Job drawing, mm, ordinate dimensions from the low corner. One solid piece. A direction names the side the tool comes from. Give positions to 0.01 mm unless a question says otherwise; leave off trailing zeros. Order: outer loops, then holes, each group sorted by start corner. A loop starts at its lowest first (then second) coordinate and runs counter-clockwise, first axis right, second up. Notation, with made-up numbers: (-5, 39) - (-1, 39) arc R18 cw to (-1, 69) - close; hole circle Ø10 at (87, -20). An arc over 180 degrees is marked (long way). Write each question's results on one line, items separated by ' | '. Start each with the question number.
1) Drop a flat-ended pin along its axis: pin 1 Ø2.5 at (x, y) = (4.5, 8.5) entering from +Z. Give the stop position or say it passes through.
2) Cut at D-D on y = 6.25. List the corners of the cut face in (x, z) (1 decimal).
3) Cut at A-A on x = 4.25. List the corners of the cut face in (y, z), plus the area to 3 significant figures.
4) Cut at C-C on z = 3.5. List the corners of the cut face in (x, y), plus the area to 3 significant figures.
5) Two-plate mould, pull along Y, no slides. Class the marked faces 3, 4, 5 and 6: +Y half, -Y half, draft (parallel to the pull), parting line (faces both ways), or undercut.
6) Tool access for the marked faces 1 and 2: list every direction of +Z, -Z, +X, -X, +Y, -Y with a clear straight run to the whole face (end or side of a thin tool).
7) Drill centre lines: line 1 along Z through (x, y) = (1.5, 2.25); line 2 along Y through (x, z) = (5.25, 10.25) (1 decimal); line 3 along X through (y, z) = (8.75, 4) (1 decimal). Where is each one in solid material? Low to high. Write a range as from..to.
8) Cut at B-B on y = 10.5. List the corners of the cut face in (x, z) (1 decimal).
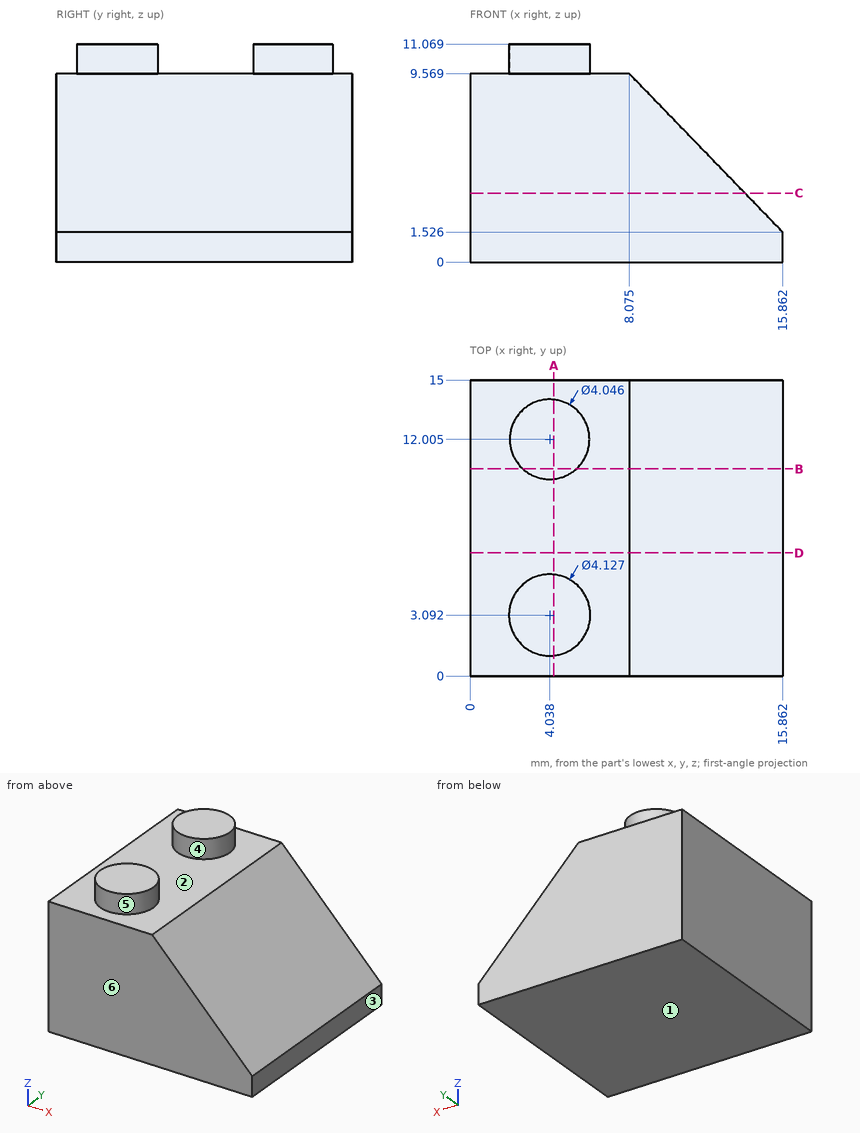
Results:
1) pin 1: z = 9.57
2) outline: (0, 0) - (15.9, 0) - (15.9, 1.5) - (8.1, 9.6) - (0, 9.6) - close
3) outline: (0, 0) - (15, 0) - (15, 9.57) - (14.02, 9.57) - (14.02, 11.07) - (9.99, 11.07) - (9.99, 9.57) - (5.14, 9.57) - (5.14, 11.07) - (1.04, 11.07) - (1.04, 9.57) - (0, 9.57) - close | area: 156 mm^2
4) outline: (0, 0) - (13.95, 0) - (13.95, 15) - (0, 15) - close | area: 209 mm^2
5) face 3: draft | face 4: undercut | face 5: undercut | face 6: -Y half
6) face 1: -Z, +X, -X, +Y, -Y | face 2: +Z
7) line 1: 0..9.57 | line 2: 1.4..4.8, 10.4..13.6 | line 3: 0..13.5
8) outline: (0, 0) - (15.9, 0) - (15.9, 1.5) - (8.1, 9.6) - (5.4, 9.6) - (5.4, 11.1) - (2.7, 11.1) - (2.7, 9.6) - (0, 9.6) - close
